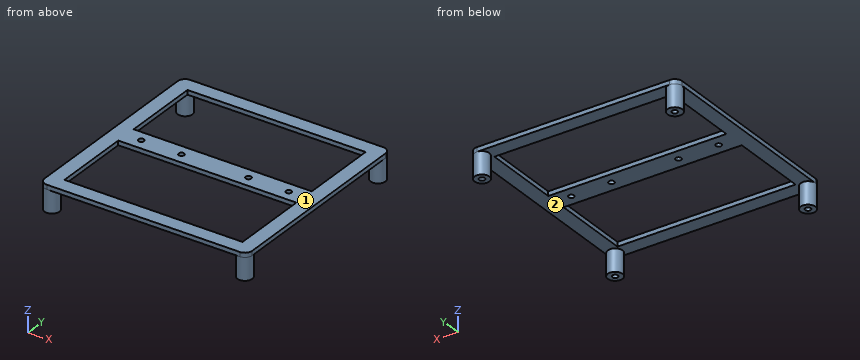
```python
from build123d import *
from build123d.topology import SkipClean

# Parameters (mm, degrees)
SKIZZE2_R                         = 3.311754822
SKIZZE2_R_2                       = 1.25
AUFSATZ_LINEAR_AUSTRAGEN1_DEPTH   = 10
SKIZZE2_R_3                       = 3.302
AUFSATZ_LINEAR_AUSTRAGEN1_2_DEPTH = 10
AUFSATZ_LINEAR_AUSTRAGEN1_3_DEPTH = 10
AUFSATZ_LINEAR_AUSTRAGEN1_4_DEPTH = 10
AUFSATZ_LINEAR_AUSTRAGEN2_DEPTH   = 2
SKIZZE4_R                         = 1.25
SCHNITT_LINEAR_AUSTRAGEN1_DEPTH   = 2


with BuildPart() as part:
    # Skizze2 → Aufsatz-Linear austragen1 (new body)
    with BuildSketch(Plane.XY):
        with Locations((-43.18, 43.18)):
            Circle(SKIZZE2_R)
        with Locations((-43.18, 43.18)):
            Circle(SKIZZE2_R_2, mode=Mode.SUBTRACT)
    extrude(amount=AUFSATZ_LINEAR_AUSTRAGEN1_DEPTH)



with BuildPart() as body_2:
    # Skizze2 → Aufsatz-Linear austragen1 2 (new body)
    with BuildSketch(Plane.XY):
        with Locations((-43.18, -43.18)):
            Circle(SKIZZE2_R_3)
        with Locations((-43.18, -43.18)):
            Circle(SKIZZE2_R_2, mode=Mode.SUBTRACT)
    extrude(amount=AUFSATZ_LINEAR_AUSTRAGEN1_2_DEPTH)


with BuildPart() as body_3:
    # Skizze2 → Aufsatz-Linear austragen1 3 (new body)
    with BuildSketch(Plane.XY):
        with Locations((43.18, -43.18)):
            Circle(SKIZZE2_R_3)
        with Locations((43.18, -43.18)):
            Circle(SKIZZE2_R_2, mode=Mode.SUBTRACT)
    extrude(amount=AUFSATZ_LINEAR_AUSTRAGEN1_3_DEPTH)


with BuildPart() as body_4:
    # Skizze2 → Aufsatz-Linear austragen1 4 (new body)
    with BuildSketch(Plane.XY):
        with Locations((43.18, 43.18)):
            Circle(SKIZZE2_R_3)
        with Locations((43.18, 43.18)):
            Circle(SKIZZE2_R_2, mode=Mode.SUBTRACT)
    extrude(amount=AUFSATZ_LINEAR_AUSTRAGEN1_4_DEPTH)


with BuildPart() as part_1:
    with SkipClean():  # the faces are left unmerged after this step: merging them gives an invalid solid
        add(part.part)

        add(body_2.part)  # Aufsatz-Linear austragen2 merges body 2

        add(body_3.part)  # Aufsatz-Linear austragen2 merges body 3

        add(body_4.part)  # Aufsatz-Linear austragen2 merges body 4
        # Skizze3 → Aufsatz-Linear austragen2 (add)
        with BuildSketch(Plane.XY.offset(10)):
            with BuildLine():
                ThreePointArc((46.482, 43.18), (45.514866591, 45.514866591), (43.18, 46.482))
                Line((43.18, 46.482), (-43.18, 46.491754822))
                ThreePointArc((-43.18, 46.491754822), (-45.521764292, 45.521764292), (-46.491754822, 43.18))
                Line((-46.491754822, 43.18), (-46.482, -43.18))
                ThreePointArc((-46.482, -43.18), (-45.514866591, -45.514866591), (-43.18, -46.482))
                Line((-43.18, -46.482), (43.18, -46.482))
                ThreePointArc((43.18, -46.482), (45.514866591, -45.514866591), (46.482, -43.18))
                Line((46.482, -43.18), (46.482, 43.18))
            make_face()
            Polygon((39.878, -39.878), (-39.877627022, -39.878), (-39.873687387, -5.000187008), (39.878, -5.000187008), align=None, mode=Mode.SUBTRACT)
            Polygon((39.878, 39.877627022), (39.878, 4.999812928), (-39.872557834, 4.999812928), (-39.868619216, 39.868619216), align=None, mode=Mode.SUBTRACT)
        extrude(amount=AUFSATZ_LINEAR_AUSTRAGEN2_DEPTH)

    # Skizze4 → Schnitt-Linear austragen1 (cut)
    with SkipClean():  # the faces are left unmerged after this step: merging them gives an invalid solid
        with BuildSketch(Plane.XY.offset(12)):
            with Locations((-33, 0)):
                Circle(SKIZZE4_R)
            with Locations((-15, 0)):
                Circle(SKIZZE4_R)
            with Locations((32.999980451, -0.035919632)):
                Circle(SKIZZE4_R)
            with Locations((14.999991114, -0.016327105)):
                Circle(SKIZZE4_R)
        extrude(amount=-SCHNITT_LINEAR_AUSTRAGEN1_DEPTH, mode=Mode.SUBTRACT)


solid = part_1.part
```
Input: part model. Units: mm. Frame: model coordinates. Face numbers are marked on the shaded views. Round coordinates to 2 decimals unless told otherwise and drop trailing zeros. Loops run counter-clockwise (first coordinate to the right, second up) from the corner with the lowest first, then second, coordinate; pieces in that order, holes last. Notation, with made-up numbers: (45, -3) -> (102, -3) arc R10 cw to (102, 12) -> close; hole circle Ø10 at (66, 47.25). An arc over 180 degrees is marked (long way). One line per item, written item: value.
(1) Mould query, pull axis Y, two halves, no side actions, for the marked faces 1 and 2. Classes: pulls with the +Y half, pulls with the -Y half, needs draft (parallel to the pull), parting line crosses it, or undercut.
Geometry check:
face 1: needs draft
face 2: undercut
(2) Pin query (flat end, axial travel): pin 1 (3 mm diameter, centred on x = 33, y = -0.04, fed in from -Z). Return the tip coordinate at first contact, or that it passes through.
Geometry check:
pin 1: z = 10
(3) Section C-C (y = -8.5). Return the cut outline in (x, z), plus the area to 3 significant figures.
Geometry check:
outline: (-46.49, 10) -> (-39.87, 10) -> (-39.87, 12) -> (-46.49, 12) -> close; (39.88, 10) -> (46.48, 10) -> (46.48, 12) -> (39.88, 12) -> close
area: 26.4 mm2
(4) Section D-D (x = -21). Return the cut outline in (y, z).
Geometry check:
outline: (-46.48, 10) -> (-39.88, 10) -> (-39.88, 12) -> (-46.48, 12) -> close; (-5, 10) -> (5, 10) -> (5, 12) -> (-5, 12) -> close; (39.87, 10) -> (46.49, 10) -> (46.49, 12) -> (39.87, 12) -> close
(5) Section A-A (z = 7.5). Return the cut outline in (x, y), plus the area to 3 significant figures.
Geometry check:
outline: circle Ø6.62 at (-43.18, 43.18); circle Ø6.6 at (-43.18, -43.18); circle Ø6.6 at (43.18, -43.18); circle Ø6.6 at (43.18, 43.18); hole circle Ø2.5 at (-43.18, -43.18); hole circle Ø2.5 at (-43.18, 43.18); hole circle Ø2.5 at (43.18, -43.18); hole circle Ø2.5 at (43.18, 43.18)
area: 118 mm2
(6) Material intervals for line 1 (Y direction, x = -43.18, z = 7.5); line 2 (Y direction, x = -19, z = 11.5); line 3 (X direction, y = -41.5, z = 11.5), sorted ascending. Write a range as [from, to].
Geometry check:
line 1: [-46.48, -44.43], [-41.93, -39.88], [39.87, 41.93], [44.43, 46.49]
line 2: [-46.48, -39.88], [-5, 5], [39.87, 46.49]
line 3: [-46.48, 46.48]
(7) Section B-B (x = -33). Return the cut outline in (y, z).
Geometry check:
outline: (-46.48, 10) -> (-39.88, 10) -> (-39.88, 12) -> (-46.48, 12) -> close; (-5, 10) -> (-1.25, 10) -> (-1.25, 12) -> (-5, 12) -> close; (1.25, 10) -> (5, 10) -> (5, 12) -> (1.25, 12) -> close; (39.87, 10) -> (46.49, 10) -> (46.49, 12) -> (39.87, 12) -> close
